Autodesk Inventor part; units mm, degrees
ref_plane "Work Plane1" through (-35.2091, 0, 0) normal (0, -0.8660254, -0.5) x (1, 0, 0)
ref_plane "YZ Plane" through (0, 0, 0) normal (1, 0, 0) x (0, 1, 0)
ref_plane "XZ Plane" through (0, 0, 0) normal (0, 1, 0) x (-1, 0, 0)
sketch "Sketch1" plane through (0, 0, 0) normal (1, 0, 0) x (0, 1, 0)
  line L0 (-19.6299, 0) -> (-9.815, 17)
  line L1 (-9.815, 17) -> (9.815, 17)
  line L2 (9.815, 17) -> (19.6299, 0)
  line L3 (19.6299, 0) -> (9.815, -17)
  line L4 (9.815, -17) -> (-9.815, -17)
  line L5 (-9.815, -17) -> (-19.6299, 0)
  point P0 (0, 0)
  point P1 (0, 0)
  dimension "d0" = 39.2598
extrude "Body" add sketch "Sketch1" along normal blind 20.7
sketch "Sketch2" plane through (0, 0, 0) normal (0, 0, 1) x (1, 0, 0)
  line L0 (0, 9.815) -> (0, 19.6299)
  line L1 (0, 19.6299) -> (20.7, 19.6299)
  line L2 (20.7, 9.815) -> (20.7, 19.6299)
  line L3 (-4.14, 0) -> (24.84, 0)
  line L4 (1.5184, 19.6299) -> (0, 17)
  line L5 (19.1816, 19.6299) -> (20.7, 17)
  dimension "d3" = 30
  dimension "d4" = 30
  dimension "d5" = 34
  dimension "d6" = 34
revolve "Chamfer1" cut sketch "Sketch2" angle 360 about axis through (-10, 0, 0) along (1, 0, 0)
sketch "Sketch3" plane through (20.7, 0, 0) normal (1, 0, 0) x (0, 0, -1)
  arc A0 (-8.5, -14.7224) -> (8.5, -14.7224) centre (0, 0) ccw
hole "Thread" at (20.7, 0, 0) direction (-1, 0, 0) diameter 17.294 end through all
chamfer "Chamfer2" distance 1.3532 angle 30 1 edges at (20.7, 0, 8.647) measured on face at (20.7, 14.1326, -0.3474)
chamfer "Chamfer3" distance 1.3532 angle 30 1 edges at (0, 0, 8.647) measured on face at (0, 14.1326, -0.3474)
ref_plane "Work Plane1" through (-35.2091, 0, 0) normal (0, -0.8660254, -0.5) x (1, 0, 0)
equation "\"d0\" = 1.1547 * SW"
equation "\"d1\" = KOH"
equation "\"d3\" = ANG1"
equation "\"d4\" = ANG2"
equation "\"d5\" = SW0"
equation "\"d6\" = SW01"
equation "\"d8\" = -0.5 * GD1 + 0.5 * NND"
equation "\"d40\" = -0.5 * GD1 + 0.5 * NND"
equation "\"d10\" = -0.5 * GD1 + 0.5 * NND"
equation "\"d41\" = -0.5 * GD1 + 0.5 * NND"
equation "\"ANG1\" = 30deg"
equation "\"ANG2\" = 30deg"
equation "\"KOH\" = 20.7"
equation "\"SW\" = 34"
equation "\"SW0\" = SW"
equation "\"SW01\" = SW"
equation "\"GUL\" = 0.541266 * PTC"
equation "\"TOA\" = 30deg"
equation "\"PTC\" = 2.5"
equation "\"E0\" = 1.155 * SW"
equation "\"GAL\" = 0.541266 * PTC"
equation "\"SD2\" = 31.4"
equation "\"WFT\" = 0"
properties part number "ANSI B18.2.4.6M - M20 x 2.5" material "Steel, Mild"
Here's how the part is built. I have some questions about the finished solid (model axes, mm). Round coordinates to 2 decimals unless told otherwise and drop trailing zeros. Loops run counter-clockwise (first coordinate to the right, second up) from the corner with the lowest first, then second, coordinate; pieces in that order, holes last. Notation, with made-up numbers: M -5,76.5 L 51,76.5 A19 ccw 51,80.5 Z; hole C 80.5,-7.5 d1. An arc over 180 degrees is marked long. Write each question's results on one line, items separated by ' | '. Start each with the question number.
(1) If I drill on probe 1 along Y at (x, z) = (12, 0); probe 2 along Z at (x, y) = (15.5, 0); probe 3 along Y at (x, z) = (5.25, -0.5), over which ranges is the centre line in solid material (lowest first)? Write a range as from..to.
(2) Will these pins go through, and if not, where does the flat tip stop? P1, Ø2, axis at x = 5, y = -11.5, coming from the -Z side; P2, Ø6, axis at x = 10.5, z = 8, coming from the +Y side; P3, Ø5, axis at y = 1, z = 7, coming from the -X side.
(3) I want a section at A-A (x = 3.75). Please give me the cut outline in (y, z) (3 decimals), then the cut area to 3 significant figures.
(4) Thinking about a two-plate mould opening in Y: for faces 1 (the conical face through (0.37, -8.86, -15.25)), 2 (the flat face through (10, 0, -17)), 3 (the cylindrical face through (10.216, 5.262, 6.862)), 4 (the conical face through (0.37, 8.78, -15.3)), which applies, pulls with the +Y half, pulls with the -Y half, needs draft (parallel to the pull), parting line crosses it, or undercut?
Solved:
1) probe 1: y = -19.63..-8.65, 8.65..19.63 | probe 2: z = -17..-8.65, 8.65..17 | probe 3: y = -19.34..-8.63, 8.63..19.34
2) P1: stops at z = -15.81 | P2: stops at y = 16.74 | P3: stops at x = 0.25
3) outline: M -19.63,0 L -9.815,-17 L 9.815,-17 L 19.63,0 L 9.815,17 L -9.815,17 Z; hole C 0,0 d17.294 | area: 766 mm²
4) face 1: pulls with the -Y half | face 2: needs draft | face 3: undercut | face 4: pulls with the +Y half
